Can you work these out from the model? Positions are in its coordinate system, mm. A direction names the side the tool comes from. Give positions to 0.01 mm unless a question says otherwise; leave off trailing zeros. Loops run counter-clockwise (first coordinate to the right, second up) from the corner with the lowest first, then second, coordinate; pieces in that order, holes last. Notation, with made-up numbers: M 77.5,28.25 L 87.5,28.25 A17 ccw 87.5,48.25 Z; hole C 85,17 d9. An arc over 180 degrees is marked long. Use CSV: the item, a comma, the result in double quotes.
from build123d import *

# Parameters (mm, degrees)
F0_W     = 88.9
F0_H     = 88.9
F1_DEPTH = 88.9
F2_T     = -2.54
F3_R     = 3.81
F4_DEPTH = 25.4


with BuildPart() as f1:
    # F0 (on Front) → F1 (new body)
    with BuildSketch(Plane.XZ):
        Rectangle(F0_W, F0_H)
    extrude(amount=F1_DEPTH)

    # F2
    f2_openings = [f1.faces().sort_by_distance(p)[0] for p in [
        (0, -44.45, 44.45),
    ]]
    offset(amount=F2_T, openings=f2_openings)

    # F3 (on face) → F4 (cut)
    with BuildSketch(Plane.YZ.offset(44.45)):
        with Locations((-44.45, 0)):
            Circle(F3_R)
    extrude(amount=-F4_DEPTH, mode=Mode.SUBTRACT)


solid = f1.part
Q1. If we mould it in two halves opening along Z, with no side actions, what happens to faces 1 (the flat face through (-44.45, -44, -1)), 2 (the cylindrical face through (43.198, -48.256, 0.168)), 3 (the flat face through (-1, -44, -44.45))? For each: released by +Z, released by -Z, zero draft, split by the parting line, or undercut.
Model answer:
face 1,"zero draft"
face 2,"undercut"
face 3,"released by -Z"
Q2. I want a section at A-A, the plane z = -13.5. Please give me the cut outline in (x, y).
Model answer:
outline,"M -44.45,-88.9 L 44.45,-88.9 L 44.45,0 L -44.45,0 Z; hole M -41.91,-86.36 L 41.91,-86.36 L 41.91,-2.54 L -41.91,-2.54 Z"
Q3. I'm going to push flat-ended pins straight in: P1, Ø5, axis at x = -22, y = -25.5, coming from the +Z side; P2, Ø7, axis at y = -44.45, z = 0, coming from the +X side. Where does each tip first touch, or does it pass through?
Model answer:
P1,"z = -41.91"
P2,"x = -41.91"
Q4. I want a section at B-B, the plane y = -44.45. Please give me the cut outline in (x, z), then the cut area to 3 significant figures.
Model answer:
outline,"M -44.45,-44.45 L 44.45,-44.45 L 44.45,-3.81 L 41.91,-3.81 L 41.91,-41.91 L -41.91,-41.91 L -41.91,44.45 L -44.45,44.45 Z; M 41.91,3.81 L 44.45,3.81 L 44.45,44.45 L 41.91,44.45 Z"
area,"645 mm2"
Q5. I want a section at C-C, the plane x = 28. Please give me the cut outline in (y, z).
Model answer:
outline,"M -88.9,-44.45 L 0,-44.45 L 0,44.45 L -2.54,44.45 L -2.54,-41.91 L -86.36,-41.91 L -86.36,44.45 L -88.9,44.45 Z"
Q6. For faces 4 (the flat face through (-1, -86.36, 2)), 5 (the flat face through (-1, 0, 1)), which set-ups out of +Z, -Z, +X, -X, +Y, -Y let a thin tool reach every point of the face, with its end or its side?
Model answer:
face 4,"+Z"
face 5,"+Z, -Z, +X, -X, +Y"
Q7. I want a section at D-D, the plane z = 0. Please give me the cut outline in (x, y), then the cut area to 3 significant figures.
Model answer:
outline,"M -44.45,-88.9 L 44.45,-88.9 L 44.45,-48.26 L 41.91,-48.26 L 41.91,-86.36 L -41.91,-86.36 L -41.91,-2.54 L 41.91,-2.54 L 41.91,-40.64 L 44.45,-40.64 L 44.45,0 L -44.45,0 Z"
area,"858 mm2"
Q8. Please list where these lines run through material, in increasing order: L1, parallel to Y at x = 11, z = -36; L2, parallel to X at y = -76.5, z = -17; L3, parallel to Z at x = 43, y = -44. Write a range as from..to.
Model answer:
L1,"-88.9..-86.36, -2.54..0"
L2,"-44.45..-41.91, 41.91..44.45"
L3,"-44.45..-3.78, 3.78..44.45"
